from build123d import *

# Parameters (mm, degrees)
SKIZZE2_R                        = 50
SKIZZE2_R_2                      = 2
AUFSATZ_LINEAR_AUSTRAGEN1_DEPTH  = 5
SCHNITT_LINEAR_AUSTRAGEN2_DEPTH  = 3
SKIZZE10_R                       = 3.5
SCHNITT_LINEAR_AUSTRAGEN3_DEPTH  = 3
SCHNITT_LINEAR_AUSTRAGEN7_DEPTH  = 3
SKIZZE27_W                       = 25
SKIZZE27_H                       = 52
SCHNITT_LINEAR_AUSTRAGEN10_DEPTH = 1
SKIZZE12_R                       = 2.5
AUFSATZ_LINEAR_AUSTRAGEN5_DEPTH  = 2
SKIZZE30_R                       = 1.25
AUFSATZ_LINEAR_AUSTRAGEN6_DEPTH  = 3
SKIZZE31_W                       = 16
SKIZZE31_H                       = 6
AUFSATZ_LINEAR_AUSTRAGEN8_DEPTH  = 5
SKIZZE32_R                       = 0.5
SCHNITT_LINEAR_AUSTRAGEN11_DEPTH = 6.5
SKIZZE35_W                       = 14
SKIZZE35_H                       = 5
AUFSATZ_LINEAR_AUSTRAGEN9_DEPTH  = 5
SKIZZE36_R                       = 0.5
SCHNITT_LINEAR_AUSTRAGEN12_DEPTH = 6.5


with BuildPart() as part:
    # Skizze2 → Aufsatz-Linear austragen1 (new body)
    with BuildSketch(Plane(origin=(0, 0, 0), x_dir=(1, 0, 0), z_dir=(0, 1, 0))):
        with Locations(Location((0, 0, 0), (0, 0, 270))):
            Circle(SKIZZE2_R)
        with Locations(Location((38.97114317, -22.5, 0), (0, 0, 270))):
            Circle(SKIZZE2_R_2, mode=Mode.SUBTRACT)
        with Locations(Location((-39.80150929, -20.996186754, 0), (0, 0, 270))):
            Circle(SKIZZE2_R_2, mode=Mode.SUBTRACT)
        with Locations(Location((0, 45, 0), (0, 0, 270))):
            Circle(SKIZZE2_R_2, mode=Mode.SUBTRACT)
        with Locations(Location((0, -35, 0), (0, 0, 270))):
            Circle(SKIZZE2_R_2, mode=Mode.SUBTRACT)
        with Locations(Location((0, -27.5, 0), (0, 0, 270))):
            Circle(SKIZZE2_R_2, mode=Mode.SUBTRACT)
    extrude(amount=AUFSATZ_LINEAR_AUSTRAGEN1_DEPTH)

    # Skizze9 → Schnitt-Linear austragen2 (cut)
    with BuildSketch(Plane(origin=(0, 5, 0), x_dir=(1, 0, 0), z_dir=(0, 1, 0))):
        with BuildLine():
            Line((-6, -39.531216002), (-6, -22.531216002))
            Line((-6, -22.531216002), (6, -22.531216002))
            Line((6, -22.531216002), (6, -39.531216002))
            ThreePointArc((6, -39.531216002), (0, 39.983959767), (-6, -39.531216002))
        make_face()
    extrude(amount=-SCHNITT_LINEAR_AUSTRAGEN2_DEPTH, mode=Mode.SUBTRACT)

    # Skizze10 → Schnitt-Linear austragen3 (cut)
    with BuildSketch(Plane.XZ):
        with Locations(Location((0, 27.5, 0), (0, 0, 270))):
            Circle(SKIZZE10_R)
        with Locations(Location((0, 35, 0), (0, 0, 270))):
            Circle(SKIZZE10_R)
        with Locations(Location((38.97114317, 22.5, 0), (0, 0, 270))):
            Circle(SKIZZE10_R)
        with Locations(Location((-39.80150929, 20.996186754, 0), (0, 0, 270))):
            Circle(SKIZZE10_R)
        with Locations(Location((0, -45, 0), (0, 0, 270))):
            Circle(SKIZZE10_R)
    extrude(amount=-SCHNITT_LINEAR_AUSTRAGEN3_DEPTH, mode=Mode.SUBTRACT)

    # Skizze11 → Schnitt-Linear austragen7 (cut)
    with BuildSketch(Plane(origin=(0, 5, 0), x_dir=(1, 0, 0), z_dir=(0, 1, 0))):
        with BuildLine():
            Line((-5.978957813, -44.319844294), (-5.978957813, -22.5))
            Line((-5.978957813, -22.5), (6, -22.531216002))
            Line((6, -22.531216002), (6, -44.317000516))
            ThreePointArc((6, -44.317000516), (22.808968791, -38.467485978), (36.005466779, -26.525514072))
            ThreePointArc((36.005466779, -26.525514072), (34.786839389, -19.762920925), (41.47114317, -18.169872981))
            ThreePointArc((41.47114317, -18.169872981), (39.210967853, 22.638462845), (5, 45))
            ThreePointArc((5, 45), (0, 40), (-5, 45))
            ThreePointArc((-5, 45), (-38.771722635, 23.382761255), (-42.13441893, -16.573796833))
            ThreePointArc((-42.13441893, -16.573796833), (-35.515787713, -18.42080512), (-36.991636347, -25.131959239))
            ThreePointArc((-36.991636347, -25.131959239), (-23.530017506, -38.030708788), (-5.978957813, -44.319844294))
        make_face()
    extrude(amount=-SCHNITT_LINEAR_AUSTRAGEN7_DEPTH, mode=Mode.SUBTRACT)

    # Skizze27 → Schnitt-Linear austragen10 (cut)
    with BuildSketch(Plane.XZ.offset(-2)):
        with Locations((21.020025154, -2.667993815)):
            Rectangle(SKIZZE27_W, SKIZZE27_H)
    extrude(amount=SCHNITT_LINEAR_AUSTRAGEN10_DEPTH, mode=Mode.SUBTRACT)

    # Skizze12 → Aufsatz-Linear austragen5 (add)
    with BuildSketch(Plane(origin=(0, 2, 0), x_dir=(1, 0, 0), z_dir=(0, 1, 0))):
        with Locations(Location((-32.155741969, 26.956104286, 0), (0, 0, 90))):
            Circle(SKIZZE12_R)
        with Locations(Location((-11.835741969, 26.956104286, 0), (0, 0, 90))):
            Circle(SKIZZE12_R)
        with Locations(Location((-32.155741969, -6.193895714, 0), (0, 0, 90))):
            Circle(SKIZZE12_R)
        with Locations(Location((-11.835741969, -6.193895714, 0), (0, 0, 90))):
            Circle(SKIZZE12_R)
    extrude(amount=AUFSATZ_LINEAR_AUSTRAGEN5_DEPTH)

    # Skizze30 → Aufsatz-Linear austragen6 (add)
    with BuildSketch(Plane(origin=(0, 4, 0), x_dir=(1, 0, 0), z_dir=(0, 1, 0))):
        with Locations(Location((-32.155741969, 26.956104286, 0), (0, 0, 270))):
            Circle(SKIZZE30_R)
        with Locations(Location((-11.835741969, 26.956104286, 0), (0, 0, 270))):
            Circle(SKIZZE30_R)
        with Locations(Location((-32.155741969, -6.193895714, 0), (0, 0, 270))):
            Circle(SKIZZE30_R)
        with Locations(Location((-11.835741969, -6.193895714, 0), (0, 0, 270))):
            Circle(SKIZZE30_R)
    extrude(amount=AUFSATZ_LINEAR_AUSTRAGEN6_DEPTH)

    # Skizze31 → Aufsatz-Linear austragen8 (add)
    with BuildSketch(Plane(origin=(0, 2, 0), x_dir=(1, 0, 0), z_dir=(0, 1, 0))):
        with Locations((-17.477480193, -13.166385762)):
            Rectangle(SKIZZE31_W, SKIZZE31_H)
        with Locations((-17.477480193, -31.166385762)):
            Rectangle(SKIZZE31_W, SKIZZE31_H)
    extrude(amount=AUFSATZ_LINEAR_AUSTRAGEN8_DEPTH)

    # Skizze32 → Schnitt-Linear austragen11 (cut)
    with BuildSketch(Plane(origin=(0, 7, 0), x_dir=(1, 0, 0), z_dir=(0, 1, 0))):
        with Locations(Location((-16.207480193, -12.166385762, 0), (0, 0, 270))):
            Circle(SKIZZE32_R)
        with Locations(Location((-13.667480193, -12.166385762, 0), (0, 0, 270))):
            Circle(SKIZZE32_R)
        with Locations(Location((-18.747480193, -12.166385762, 0), (0, 0, 270))):
            Circle(SKIZZE32_R)
        with Locations(Location((-21.287480193, -12.166385762, 0), (0, 0, 270))):
            Circle(SKIZZE32_R)
        with Locations(Location((-16.207480193, -32.166385762, 0), (0, 0, 270))):
            Circle(SKIZZE32_R)
        with Locations(Location((-13.667480193, -32.166385762, 0), (0, 0, 270))):
            Circle(SKIZZE32_R)
        with Locations(Location((-11.127480193, -32.166385762, 0), (0, 0, 270))):
            Circle(SKIZZE32_R)
        with Locations(Location((-18.747480193, -32.166385762, 0), (0, 0, 270))):
            Circle(SKIZZE32_R)
        with Locations(Location((-21.287480193, -32.166385762, 0), (0, 0, 270))):
            Circle(SKIZZE32_R)
        with Locations(Location((-23.827480193, -32.166385762, 0), (0, 0, 270))):
            Circle(SKIZZE32_R)
    extrude(amount=-SCHNITT_LINEAR_AUSTRAGEN11_DEPTH, mode=Mode.SUBTRACT)

    # Skizze35 → Aufsatz-Linear austragen9 (add)
    with BuildSketch(Plane(origin=(0, 2, 0), x_dir=(1, 0, 0), z_dir=(0, 1, 0))):
        with Locations((0, 35.385800952)):
            Rectangle(SKIZZE35_W, SKIZZE35_H)
    extrude(amount=AUFSATZ_LINEAR_AUSTRAGEN9_DEPTH)

    # Skizze36 → Schnitt-Linear austragen12 (cut)
    with BuildSketch(Plane(origin=(0, 7, 0), x_dir=(1, 0, 0), z_dir=(0, 1, 0))):
        with Locations(Location((1.118435078, 35.339246481, 0), (0, 0, 270))):
            Circle(SKIZZE36_R)
        with Locations(Location((3.658435078, 35.339246481, 0), (0, 0, 270))):
            Circle(SKIZZE36_R)
        with Locations(Location((-1.421564922, 35.339246481, 0), (0, 0, 270))):
            Circle(SKIZZE36_R)
        with Locations(Location((-3.961564922, 35.339246481, 0), (0, 0, 270))):
            Circle(SKIZZE36_R)
    extrude(amount=-SCHNITT_LINEAR_AUSTRAGEN12_DEPTH, mode=Mode.SUBTRACT)


solid = part.part
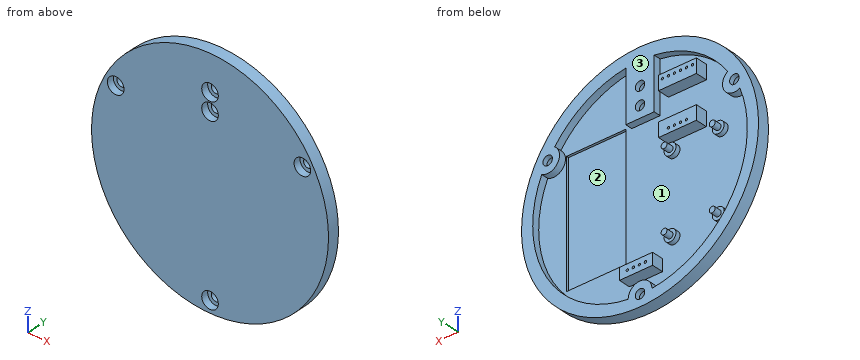
Read the model definition and answer for the solid it produces. Units are mm, in the model's axes. Face numbers are marked on the shaded views. Coordinates: 2 decimals unless noted, no trailing zeros. Loops run counter-clockwise (first coordinate to the right, second up) from the corner with the lowest first, then second, coordinate; pieces in that order, holes last. Notation, with made-up numbers: (74, 24) -> (92, 24) arc R20 ccw to (92, 34) -> close; hole circle Ø2 at (11.5, -25.5). An arc over 180 degrees is marked (long way). Write item = value, one per line. Start each with the question number.
1) The part is cut by section A-A, the plane z = 0. Determine the outline of the cut face in (x, y).
2) Find the intervals of material crossed by L1, parallel to X at y = 3.5, z = 26; L2, parallel to X at y = 3.5, z = 11 (3 decimals); L3, parallel to Y at x = 1, z = -1.5, in increasing order. Write a range as from..to.
3) Given P1, Ø10, axis at x = 35.5, z = 39, coming from the +Y side; P2, Ø4, axis at x = -20, y = 5, coming from the +Z side; P3, Ø0.8, axis at x = -21.5, z = 12.5, coming from the +Y side; P4, Ø12, axis at x = -30, z = -3.5, coming from the +Y side, each flat-ended and moving along its own axis, determine where each tip first touches the part or whether it passes through.
4) The mould has two halves that part along X. Classify the marked faces 1, 2 and 3: pulls with the +X half, pulls with the -X half, needs draft (parallel to the pull), parting line crosses it, or undercut.
Result:
q1.outline = (-50, 0) -> (50, 0) -> (50, 5) -> (45.28, 5) -> (45.28, 2) -> (33.52, 2) -> (33.52, 1) -> (8.52, 1) -> (8.52, 2) -> (-45.28, 2) -> (-45.28, 5) -> (-50, 5) -> close
q2.L1 = -42.71..-36.39, -5.98..-1.32, 1.32..6, 35.4..42.71
q2.L2 = -48.775..-43.92, -25.477..-9.477, 43.92..48.775
q2.L3 = 0..2
q3.P1 = 5
q3.P2 = 46.65
q3.P3 = 7
q3.P4 = 2
q4.face_1 = undercut
q4.face_2 = undercut
q4.face_3 = needs draft
